For this review, take the finished solid that the model builds, in its own axes (mm). A direction names the side the tool comes from. Coordinates: 2 decimals unless noted, no trailing zeros. Write each loop counter-clockwise with the first axis right and the second up, starting at its lowest first coordinate (ties: lowest second). Pieces come first, ordered by that corner, then holes.
1) We need section A-A on z = 0.5. Write out the cut boundary in (x, y), then the cut area to 3 significant figures.
2) For faces 1 (the face through (26.746, 3.115, -0.311)), 2 (the face through (11, 0, 0)), 3 (the face through (30.031, -4.332, -0.764)), 4 (the face through (16, -2.5, 1)), 5 (the face through (16, 2.5, 1)), list the 3-axis set-ups (+Z, -Z, +X, -X, +Y, -Y) from which the entire face can be reached by the end or side of a thin tool; tool diameter is ignored.
3) We need section B-B on y = 1.5. Give the number of separate pieces and of enclosed holes in the cut face, then the cut area to 3 significant figures.
4) We need section C-C on x = 12. Write out the cut boundary in (y, z), then the cut area to 3 significant figures.
5) Mouldability with a two-part tool opening along Y and no side actions: class faces 6 (the face through (35.847, 0.766, 2.986)), 7 (the face through (0, 0, 10)), 8 (the face through (-2.5, 0.1, 1)), 9 (the face through (33, -4.5, 3)) as pulls with the +Y half, pulls with the -Y half, needs draft (parallel to the pull), parting line crosses it, or undercut.
6) To check wall thickness, follow line 1 along Y through (x, z) = (34, 3.1); line 2 along Z through (x, y) = (36, 3.25); line 3 along Y through (x, z) = (11.5, 1.75). State the ranges of each line that lie inside material, in increasing order.
7) Insertion check: P1, Ø4, axis at x = 10, y = -0.5, coming from the -Z side; P2, Ø2, axis at x = 21.5, y = 1.5, coming from the +Z side; P3, Ø2, axis at x = 20, z = 1, coming from the +Y side. Each pin has a flat end and moves straight along its axis. Give the tip position at first contact, or say it passes through.
8) We need section D-D on z = 6.5. Write out the cut boundary in (x, y), then the cut area to 3 significant figures.
from build123d import *

# Parameters (mm, degrees)
BOSS_EXTRUDE1_DEPTH = 2
SKETCH2_R           = 2
BOSS_EXTRUDE2_DEPTH = 8
SKETCH5_R           = 3.5
CUT_EXTRUDE2_DEPTH  = 5
BOSS_EXTRUDE3_DEPTH = 2
CUT_EXTRUDE1_DEPTH  = 5.5
SKETCH6_R           = 2
CUT_EXTRUDE3_DEPTH  = 11


with BuildPart() as part:
    # Sketch1 → Boss-Extrude1 (new body)
    with BuildSketch(Plane.XY):
        with BuildLine():
            Line((0, -2.5), (34, -2.5))
            ThreePointArc((34, -2.5), (36.5, 0), (34, 2.5))
            Line((34, 2.5), (0, 2.5))
            ThreePointArc((0, 2.5), (-2.5, 0), (0, -2.5))
        make_face()
    extrude(amount=BOSS_EXTRUDE1_DEPTH)

    # Sketch2 → Boss-Extrude2 (add)
    with BuildSketch(Plane.XY.offset(2)):
        Circle(SKETCH2_R)
    extrude(amount=BOSS_EXTRUDE2_DEPTH)

    # Sketch5 → Cut-Extrude2 (cut, symmetric)
    with BuildSketch(Plane(origin=(0, 0, 0), x_dir=(-1, 0, 0), z_dir=(0, 0, -1))):
        with Locations((-34, 0)):
            Circle(SKETCH5_R)
    extrude(amount=CUT_EXTRUDE2_DEPTH, both=True, mode=Mode.SUBTRACT)

    # Sketch3 → Boss-Extrude3 (add)
    with BuildSketch(Plane(origin=(0, 0, 0), x_dir=(-1, 0, 0), z_dir=(0, 0, -1))):
        with BuildLine():
            Line((-34, -4.5), (-31.853983948, -4.5))
            ThreePointArc((-31.853983948, -4.5), (-29.476132044, -4.213177664), (-27.234684348, -3.369164065))
            Line((-27.234684348, -3.369164065), (-26.000115193, -2.726167187))
            ThreePointArc((-26.000115193, -2.726167187), (-25.551825654, -2.557364467), (-25.076255273, -2.5))
            Line((-25.076255273, -2.5), (-25.076255273, 2.5))
            ThreePointArc((-25.076255273, 2.5), (-25.551825654, 2.557364467), (-26.000115193, 2.726167187))
            Line((-26.000115193, 2.726167187), (-27.234684348, 3.369164065))
            ThreePointArc((-27.234684348, 3.369164065), (-29.476132044, 4.213177664), (-31.853983948, 4.5))
            Line((-31.853983948, 4.5), (-34, 4.5))
            ThreePointArc((-34, 4.5), (-38.5, 0), (-34, -4.5))
        make_face()
    boss_extrude3 = extrude(amount=BOSS_EXTRUDE3_DEPTH)

    # Sketch4 → Cut-Extrude1 (cut, symmetric)
    with BuildSketch(Plane(origin=(0, 0, 0), x_dir=(1, 0, 0), z_dir=(0, 1, 0))):
        with BuildLine():
            Line((31.853983948, 2), (31.853983948, 3.174344261))
            Line((31.853983948, 3.174344261), (24.383890118, 3.174344261))
            Line((24.383890118, 3.174344261), (25.076255273, 0))
            add(Edge.make_bspline(
                [(31.853983948, 2), (29.962456018, 2.02071595), (29.16990367, 1.605069608), (25.966821868, 0.283607958), (25.076255273, 0)],
                knots=[0, 0, 0, 0, 0.608348739, 1, 1, 1, 1], degree=3))
        make_face()
    cut_extrude1 = extrude(amount=CUT_EXTRUDE1_DEPTH, both=True, mode=Mode.SUBTRACT)

    # Mirror1: Boss-Extrude3, Cut-Extrude1 across plane
    add(boss_extrude3.mirror(Plane.XY.offset(1)))
    add(cut_extrude1.mirror(Plane.XY.offset(1)), mode=Mode.SUBTRACT)

    # Sketch6 → Cut-Extrude3 (cut, symmetric)
    with BuildSketch(Plane(origin=(0, 0, -2), x_dir=(-1, 0, 0), z_dir=(0, 0, -1))):
        with Locations(Location((-34, 0, 0), (0, 0, 180))):
            Circle(SKETCH6_R)
    extrude(amount=CUT_EXTRUDE3_DEPTH, both=True, mode=Mode.SUBTRACT)


solid = part.part
Result:
1. outline: (0, -2.5) - (31.55, -2.5) arc R3.5 cw to (31.55, 2.5) - (0, 2.5) arc R2.5 ccw to start
1. area: 164 mm2
2. face 1: +Z, -Z, -X, +Y
2. face 2: -Z, -X, +Y, -Y
2. face 3: +Z, -Z, -X, -Y
2. face 4: +X, -X, -Y
2. face 5: +X, -X, +Y
3. separate pieces: 3
3. enclosed holes: 0
3. area: 118 mm2
4. outline: (-2.5, 0) - (2.5, 0) - (2.5, 2) - (-2.5, 2) - close
4. area: 10.0 mm2
5. face 6: undercut
5. face 7: needs draft
5. face 8: parting line crosses it
5. face 9: pulls with the -Y half
6. line 1: y = -4.5 to -2, 2 to 4.5
6. line 2: z = -2 to 0, 2 to 4
6. line 3: y = -2.5 to 2.5
7. P1: stops at z = 0
7. P2: stops at z = 2
7. P3: stops at y = 2.5
8. outline: circle Ø4 at (0, 0)
8. area: 12.6 mm2
